Geometry check sheet. Reference: the model listing, model coordinates, mm. A direction names the side the tool comes from. Coordinates: 2 decimals unless noted, no trailing zeros. Order: outer loops, then holes, each group sorted by start corner. A loop starts at its lowest first (then second) coordinate and runs counter-clockwise, first axis right, second up. Notation, with made-up numbers: M 73.25,-1 L 111.25,-1 A7 ccw 111.25,6 Z; hole C -17.5,-24.5 d9. An arc over 180 degrees is marked long. One line per item, written item: value. Start each with the question number.
1) Sectioned sample at A-A, the plane y = 9.75. Enter the section's corners in (x, z), then the cut area to 3 significant figures.
2) Access from +Z, -Z, +X, -X, +Y, -Y to the whole of each face (thin tool, end or side, straight path). Record for faces 5 (the cylindrical face through (65, -9, 0)), 6 (the cylindrical face through (-1, -3, 0)), 7 (the flat face through (-67, -11, 0)), 8 (the cylindrical face through (65, 9, 0)), 9 (the flat face through (-67, 11, 0)).
3) Draft check along X on faces 1 (the cylindrical face through (-65, -9, 0)), 2 (the flat face through (67, -11, 0)), 3 (the cylindrical face through (-65, 9, 0)), 4 (the flat face through (-73, 0, 0)). Enter one of: pulls with the +X half, pulls with the -X half, needs draft (parallel to the pull), parting line crosses it, or undercut.
4) Sectioned sample at C-C, the plane x = -67. Enter the section's corners in (y, z).
5) Go/stop test with flat-tipped pins: P1, Ø8, axis at x = 0.5, z = 4.5, coming from the +Y side; P2, Ø3, axis at x = 26, z = 2, coming from the -Y side; P3, Ø3, axis at x = -42.5, z = -3.5, coming from the -Y side. Record where each tip stops, or that it passes through.
6) Sectioned sample at B-B, the plane z = 0. Enter the section's corners in (x, y), then the cut area to 3 significant figures.
7) Sectioned sample at D-D, the plane y = 0. Enter the section's corners in (x, z).
8) Thickness scan on L1, parallel to X at y = 0.75, z = 4.5; L2, parallel to X at y = -5, z = -0.5; L3, parallel to Z at x = -34.5, y = -1. Record the ranges inside material, lowest first. Write a range as from..to.
```python
from build123d import *

# Parameters (mm, degrees)
SKETCH_2_R      = 2
EXTRUDE_1_DEPTH = 11


with BuildPart() as part:
    # 草图1 → 旋转1 (revolve)
    with BuildSketch(Plane.XY):
        with BuildLine():
            Line((73, 0), (73, 4.5))
            ThreePointArc((73, 4.5), (66.132008426, 7.449603387), (60.126136458, 3))
            Line((60.126136458, 3), (-60.126136458, 3))
            ThreePointArc((-60.126136458, 3), (-66.132008426, 7.449603387), (-73, 4.5))
            Line((-73, 4.5), (-73, 0))
            Line((-73, 0), (73, 0))
        make_face()
    revolve(axis=Axis((-104.662512522, 0, 0), (1, 0, 0)))

    # 草图2 → 凸台-拉伸1 (add, symmetric)
    with BuildSketch(Plane(origin=(0, 0, 0), x_dir=(1, 0, 0), z_dir=(0, 1, 0))):
        with Locations(Location((67, 0, 0), (0, 0, 90))):
            Circle(SKETCH_2_R)
    extrude_1 = extrude(amount=EXTRUDE_1_DEPTH, both=True)

    # 镜向1: 凸台-拉伸1 across plane
    add(extrude_1.mirror(Plane(origin=(0, 0, 0), x_dir=(0, 0, 1), z_dir=(1, 0, 0))))


solid = part.part
```
Final values:
1. outline: C -67,0 d4; C 67,0 d4
1. area: 25.1 mm^2
2. face 5: -Y
2. face 6: none
2. face 7: +Z, -Z, +X, -X, -Y
2. face 8: +Y
2. face 9: +Z, -Z, +X, -X, +Y
3. face 1: undercut
3. face 2: needs draft
3. face 3: undercut
3. face 4: pulls with the -X half
4. outline: M -11,-2 L -7.23,-2 A7.5 ccw 7.23,-2 L 11,-2 L 11,2 L 7.23,2 A7.5 ccw -7.23,2 L -11,2 Z
5. P1: stops at y = 2.96
5. P2: stops at y = -2.96
5. P3: stops at y = -2.24
6. outline: M -73,-4.5 A7.5 ccw -69,-7.23 L -69,-11 L -65,-11 L -65,-7.23 A7.5 ccw -60.13,-3 L 60.13,-3 A7.5 ccw 65,-7.23 L 65,-11 L 69,-11 L 69,-7.23 A7.5 ccw 73,-4.5 L 73,4.5 A7.5 ccw 69,7.23 L 69,11 L 65,11 L 65,7.23 A7.5 ccw 60.13,3 L -60.13,3 A7.5 ccw -65,7.23 L -65,11 L -69,11 L -69,7.23 A7.5 ccw -73,4.5 Z
6. area: 1,110 mm^2
7. outline: M -73,-4.5 A7.5 ccw -60.13,-3 L 60.13,-3 A7.5 ccw 73,-4.5 L 73,4.5 A7.5 ccw 60.13,3 L -60.13,3 A7.5 ccw -73,4.5 Z
8. L1: x = -72.95..-61.05, 61.05..72.95
8. L2: x = -72.57..-61.43, 61.43..72.57
8. L3: z = -2.83..2.83
